Geometry check sheet. Reference: the model listing, model coordinates, mm. A direction names the side the tool comes from. Coordinates: 2 decimals unless noted, no trailing zeros. One line per item, written item: value.
from build123d import *

# Parameters (mm, degrees)
ESQUISSE1_R                     = 33
BOSS_EXTRU_1_DEPTH              = 3
ESQUISSE2_R                     = 33
BOSS_EXTRU_2_DEPTH              = 5
CONG_1_R                        = 2
ESQUISSE3_R                     = 22
BOSS_EXTRU_3_DEPTH              = 6
CHANFREIN1_SIZE                 = 3
CONG_2_R                        = 2
CHANFREIN2_SIZE                 = 3
ESQUISSE5_R                     = 27.000000000000004
ESQUISSE5_R_2                   = 24.000000000000004
ENL_V_DE_MAT_EXTRU_MINCE1_DEPTH = 4
ENL_V_MAT_EXTRU_1_DEPTH         = 53.44951392438422
ENL_V_MAT_EXTRU_1_DEPTH_BACK    = 53.44951392438422
ESQUISSE7_R                     = 23.930546597488352
ESQUISSE7_R_2                   = 21.930546597488352
ESQUISSE7_R_3                   = 8.12388129582667
ESQUISSE7_R_4                   = 6.123881295826671
ENL_V_DE_MAT_EXTRU_MINCE2_DEPTH = 2
CHANFREIN3_SIZE                 = 2
CHANFREIN4_SIZE2                = 2
CHANFREIN4_SIZE                 = 5.494954839
CHANFREIN5_SIZE                 = 4
CHANFREIN5_SIZE2                = 6.928203230275547
CHANFREIN6_SIZE                 = 4
CHANFREIN6_SIZE2                = 6.928203230275547


with BuildPart() as part:
    # Esquisse1 → Boss.-Extru.1 (new body)
    with BuildSketch(Plane.XY):
        Circle(ESQUISSE1_R)
        with BuildLine():
            Line((-10.675959520705847, -4.138404077932739), (-14.568869579057516, -5.436040764049933))
            ThreePointArc((-14.568869579057516, -5.436040764049933), (-15.362379148266376, 2.4082788262388735), (-12.206501566003407, 9.633473907119715))
            Line((-12.206501566003407, 9.633473907119715), (-8.89742874273069, 7.206820503386352))
            ThreePointArc((-8.89742874273069, 7.206820503386352), (-11.311848311745987, 1.773298556941165), (-10.675959520705847, -4.138404077932739))
        make_face(mode=Mode.SUBTRACT)
        with BuildLine():
            Line((14.568869579057514, 5.436040764049934), (10.675959520705844, 4.138404077932738))
            ThreePointArc((10.675959520705844, 4.138404077932738), (11.311848311745983, -1.7732985569411592), (8.897428742730693, -7.206820503386345))
            Line((8.897428742730693, -7.206820503386345), (12.206501566003409, -9.633473907119711))
            ThreePointArc((12.206501566003409, -9.633473907119711), (15.362379148266374, -2.4082788262388677), (14.568869579057514, 5.436040764049934))
        make_face(mode=Mode.SUBTRACT)
    extrude(amount=BOSS_EXTRU_1_DEPTH)

    # Esquisse2 → Boss.-Extru.2 (add)
    with BuildSketch(Plane.XY.offset(3)):
        Circle(ESQUISSE2_R)
        with BuildLine():
            Line((-12.102216214336107, -9.764162160751955), (-8.819426211517364, -7.302069658637931))
            ThreePointArc((-8.819426211517364, -7.302069658637931), (-11.449834531594213, -0.061556470926751), (-8.897428742730693, 7.206820503386354))
            Line((-8.897428742730693, 7.206820503386354), (-12.206501566003409, 9.633473907119713))
            ThreePointArc((-12.206501566003409, 9.633473907119713), (-15.549775280898679, -0.08359852601843287), (-12.102216214336107, -9.764162160751955))
        make_face(mode=Mode.SUBTRACT)
        with BuildLine():
            Line((12.102216214336359, 9.76416216075164), (8.819426211517387, 7.302069658637905))
            ThreePointArc((8.819426211517387, 7.302069658637905), (11.449834531594213, 0.06155647092658078), (8.897428742730495, -7.206820503386595))
            Line((8.897428742730495, -7.206820503386595), (12.206501566003364, -9.63347390711977))
            ThreePointArc((12.206501566003364, -9.63347390711977), (15.54977528089868, 0.0835985260181948), (12.102216214336359, 9.76416216075164))
        make_face(mode=Mode.SUBTRACT)
    extrude(amount=BOSS_EXTRU_2_DEPTH)

    # Congé1
    cong_1_edges = [part.edges().sort_by_distance(p)[0] for p in [
        (-12.622414549881682, -4.787222420991336, 3),
        (12.622414549881679, 4.787222420991336, 3),
    ]]
    fillet(cong_1_edges, radius=CONG_1_R)

    # Esquisse3 → Boss.-Extru.3 (add)
    with BuildSketch(Plane.XY.offset(8)):
        Circle(ESQUISSE3_R)
    extrude(amount=BOSS_EXTRU_3_DEPTH)

    # Esquisse4 → Révolution3 (revolve)
    with BuildSketch(Plane(origin=(0, 0, 0), x_dir=(1, 0, 0), z_dir=(0, 1, 0))):
        with BuildLine():
            Line((0, -13.999999999999998), (0, -23.936405555224336))
            ThreePointArc((0, -23.936405555224336), (-0.8193291269458294, -23.773207312008758), (-1.5135934632740111, -23.308523638793037))
            ThreePointArc((-1.5135934632740111, -23.308523638793037), (-7.677772539936917, -18.09763553075605), (-14.631896612797249, -14))
            Line((-14.631896612797249, -14), (0, -13.999999999999998))
        make_face()
    revolve(axis=Axis((0, 0, 13.999999999999998), (0, 0, 1)))

    # Chanfrein1
    chanfrein1_edges = [part.edges().sort_by_distance(p)[0] for p in [
        (-33, 4.04e-15, 0),
    ]]
    chamfer(chanfrein1_edges, length=CHANFREIN1_SIZE)

    # Congé2
    cong_2_edges = [part.edges().sort_by_distance(p)[0] for p in [
        (-22, 1.246e-14, 8),
    ]]
    fillet(cong_2_edges, radius=CONG_2_R)

    # Chanfrein2
    chanfrein2_edges = [part.edges().sort_by_distance(p)[0] for p in [
        (-22, 1.246e-14, 14),
    ]]
    chamfer(chanfrein2_edges, length=CHANFREIN2_SIZE)

    # Esquisse5 → Enlèv. de mat.-Extru.-Mince1 (cut)
    with BuildSketch(Plane.XY.offset(8)):
        Circle(ESQUISSE5_R)
        Circle(ESQUISSE5_R_2, mode=Mode.SUBTRACT)
    extrude(amount=-ENL_V_DE_MAT_EXTRU_MINCE1_DEPTH, mode=Mode.SUBTRACT)

    # Esquisse6 → Enlèv. mat.-Extru.1 (cut, two sides: drawn at the far end of the back side and taken through both)
    with BuildSketch(Plane(origin=(0, 0, 0), x_dir=(-1, 0, 0), z_dir=(0, 0, -1)).offset(-ENL_V_MAT_EXTRU_1_DEPTH_BACK)):
        with BuildLine():
            Line((17.457714452044502, -21.891281509104868), (21.744690267234997, -27.266979149873006))
            Line((21.744690267234997, -27.266979149873006), (10.757517205682898, -34.42702004009948))
            Line((10.757517205682898, -34.42702004009948), (-4.348149134028366, -34.02756682996412))
            add(Edge.make_bspline(
                [(17.457714452044502, -21.891281509104868), (8.150142920234186, -30.55152022572505), (-4.348149134028366, -34.02756682996412)],
                knots=[0, 0, 0, 1, 1, 1], degree=2))
        make_face()
        with BuildLine():
            Line((28, 0), (34.87577535736795, 0))
            Line((34.87577535736795, 0), (33.62333038597071, -13.05433027879381))
            Line((33.62333038597071, -13.05433027879381), (23.89279637742328, -24.61536078399858))
            add(Edge.make_bspline(
                [(28, 0), (28.967671344187806, -12.676522970367387), (23.89279637742328, -24.61536078399858)],
                knots=[0, 0, 0, 1, 1, 1], degree=2))
        make_face()
        with BuildLine():
            Line((-6.230586150776911, -27.29798154109103), (-7.760590104972264, -34.00136685488099))
            Line((-7.760590104972264, -34.00136685488099), (-20.208925843844458, -29.875461527982615))
            Line((-20.208925843844458, -29.875461527982615), (-29.314849661478412, -17.816321017099597))
            add(Edge.make_bspline(
                [(-6.230586150776911, -27.29798154109103), (-18.80460935527342, -25.420599613673357), (-29.314849661478412, -17.816321017099597)],
                knots=[0, 0, 0, 1, 1, 1], degree=2))
        make_face()
        with BuildLine():
            Line((-25.22712830126781, -12.148744695291473), (-31.421987840946983, -15.132031816678607))
            Line((-31.421987840946983, -15.132031816678607), (-35.95763554599567, -2.827071136940631))
            Line((-35.95763554599567, -2.827071136940631), (-32.20687047987901, 11.810977908358138))
            add(Edge.make_bspline(
                [(-25.22712830126781, -12.148744695291473), (-31.59910724213477, -1.1474490067937917), (-32.20687047987901, 11.810977908358138)],
                knots=[0, 0, 0, 1, 1, 1], degree=2))
        make_face()
        with BuildLine():
            Line((-25.22712830126764, 12.148744695291825), (-31.42198784094677, 15.132031816679044))
            Line((-31.42198784094677, 15.132031816679044), (-24.629512279918224, 26.350161481959308))
            Line((-24.629512279918224, 26.350161481959308), (-10.846460926500809, 32.54436956877975))
            add(Edge.make_bspline(
                [(-25.22712830126764, 12.148744695291825), (-20.598832871349522, 23.98975410589561), (-10.846460926500809, 32.54436956877975)],
                knots=[0, 0, 0, 1, 1, 1], degree=2))
        make_face()
        with BuildLine():
            Line((-6.230586150776541, 27.297981541091115), (-7.760590104971805, 34.00136685488109))
            Line((-7.760590104971805, 34.00136685488109), (5.245136083428826, 35.68518505960543))
            Line((5.245136083428826, 35.68518505960543), (18.68155493201407, 28.77118715975353))
            add(Edge.make_bspline(
                [(-6.230586150776541, 27.297981541091115), (5.9127827911769995, 31.062183075042935), (18.68155493201407, 28.77118715975353)],
                knots=[0, 0, 0, 1, 1, 1], degree=2))
        make_face()
        with BuildLine():
            Line((17.457714452044808, 21.891281509104626), (21.74469026723538, 27.266979149872704))
            Line((21.74469026723538, 27.266979149872704), (31.17008999467649, 18.148536442251835))
            Line((31.17008999467649, 18.148536442251835), (34.14197889244976, 3.3327139941706876))
            add(Edge.make_bspline(
                [(17.457714452044808, 21.891281509104626), (27.971952413158835, 14.744154635620854), (34.14197889244976, 3.3327139941706876)],
                knots=[0, 0, 0, 1, 1, 1], degree=2))
        make_face()
    extrude(amount=ENL_V_MAT_EXTRU_1_DEPTH + ENL_V_MAT_EXTRU_1_DEPTH_BACK, mode=Mode.SUBTRACT)

    # Esquisse7 → Enlèv. de mat.-Extru.-Mince2 (cut)
    # profile 1 of 2: a face of its own
    with BuildSketch(Plane(origin=(0, 0, 0), x_dir=(-1, 0, 0), z_dir=(0, 0, -1))):
        Circle(ESQUISSE7_R)
        Circle(ESQUISSE7_R_2, mode=Mode.SUBTRACT)
    # profile 2 of 2: a face of its own
    with BuildSketch(Plane(origin=(0, 0, 0), x_dir=(-1, 0, 0), z_dir=(0, 0, -1))):
        Circle(ESQUISSE7_R_3)
        Circle(ESQUISSE7_R_4, mode=Mode.SUBTRACT)
    extrude(amount=-ENL_V_DE_MAT_EXTRU_MINCE2_DEPTH, mode=Mode.SUBTRACT)

    # Chanfrein3
    chanfrein3_edges = [part.edges().sort_by_distance(p)[0] for p in [
        (6.123881295826671, 7.5e-16, 0),
    ]]
    chamfer(chanfrein3_edges, length=CHANFREIN3_SIZE - 0.0001)  # a hair under: the kernel refuses the full size

    # Chanfrein4
    chanfrein4_edges = [part.edges().sort_by_distance(p)[0] for p in [
        (21.930546597488352, 2.69e-15, 0),
    ]]
    chanfrein4_side = [part.faces().sort_by_distance(p)[0] for p in [
        (21.890546597488353, 2.68e-15, 0),
    ]]
    chamfer(chanfrein4_edges, length=CHANFREIN4_SIZE - 0.0001, length2=CHANFREIN4_SIZE2 - 0.0001, reference=chanfrein4_side[0])  # a hair under: the kernel refuses the full size

    # Chanfrein5
    chanfrein5_edges = [part.edges().sort_by_distance(p)[0] for p in [
        (10.551965154367052, -8.420147205253029, 0),
    ]]
    chanfrein5_side = [part.faces().sort_by_distance(p)[0] for p in [
        (15.970820194651594, 1.96e-15, 0),
    ]]
    chamfer(chanfrein5_edges, length=CHANFREIN5_SIZE, length2=CHANFREIN5_SIZE2, reference=chanfrein5_side[0])

    # Chanfrein6
    chanfrein6_edges = [part.edges().sort_by_distance(p)[0] for p in [
        (-10.55196515436705, 8.420147205253034, 0),
    ]]
    chanfrein6_side = [part.faces().sort_by_distance(p)[0] for p in [
        (10.37156741301878, -3.6198944951765126, 0),
    ]]
    chamfer(chanfrein6_edges, length=CHANFREIN6_SIZE, length2=CHANFREIN6_SIZE2, reference=chanfrein6_side[0])


solid = part.part
(1) Release check for a two-part mould opening along Y. For faces 1 (the face through (27.45, -13.22, 4.06)), 2 (the face through (-15.193, -11.65, 13.854)), 3 (the face through (4.15, -32.74, 5.47)) record: pulls with the +Y half, pulls with the -Y half, needs draft (parallel to the pull), parting line crosses it, or undercut.
Reply:
face 1: undercut
face 2: parting line crosses it
face 3: pulls with the -Y half
(2) Go/stop test with flat-tipped pins: pin 1 Ø12 at (y, z) = (-1.5, 14.5) entering from -X; pin 2 Ø11.5 at (x, y) = (8, -9) entering from +Z; pin 3 Ø2 at (x, z) = (8, 16) entering from -Y. Record where each tip stops, or that it passes through.
Reply:
pin 1: x = -22.64
pin 2: z = 19.12
pin 3: y = -9.95
(3) Material ranges on probe 1 along Y at (x, z) = (0, 6.45); probe 2 along Y at (x, z) = (-0.5, 6.75); probe 3 along Z at (x, y) = (-27, -8.5), recorded low to high. Write a range as from..to.
Reply:
probe 1: -32.63..-27, -24..24, 27..28.82
probe 2: -32.44..-27, -23.99..23.99, 27..28.91
probe 3: 0..8
(4) Access from +Z, -Z, +X, -X, +Y, -Y to the whole of each face (thin tool, end or side, straight path). Record for faces 4 (the face through (2, 6, 2)), 5 (the face through (10, -11, 14)), 6 (the face through (-11.299, 1.856, 3.944)).
Reply:
face 4: -Z
face 5: +Z
face 6: none
